Print and shaded views of the part. All mm, measured from the part's lowest x, y and z. A direction names the side the tool comes from. Coordinates: 2 decimals unless noted, no trailing zeros. Order: outer loops, then holes, each group sorted by start corner. A loop starts at its lowest first (then second) coordinate and runs counter-clockwise, first axis right, second up.
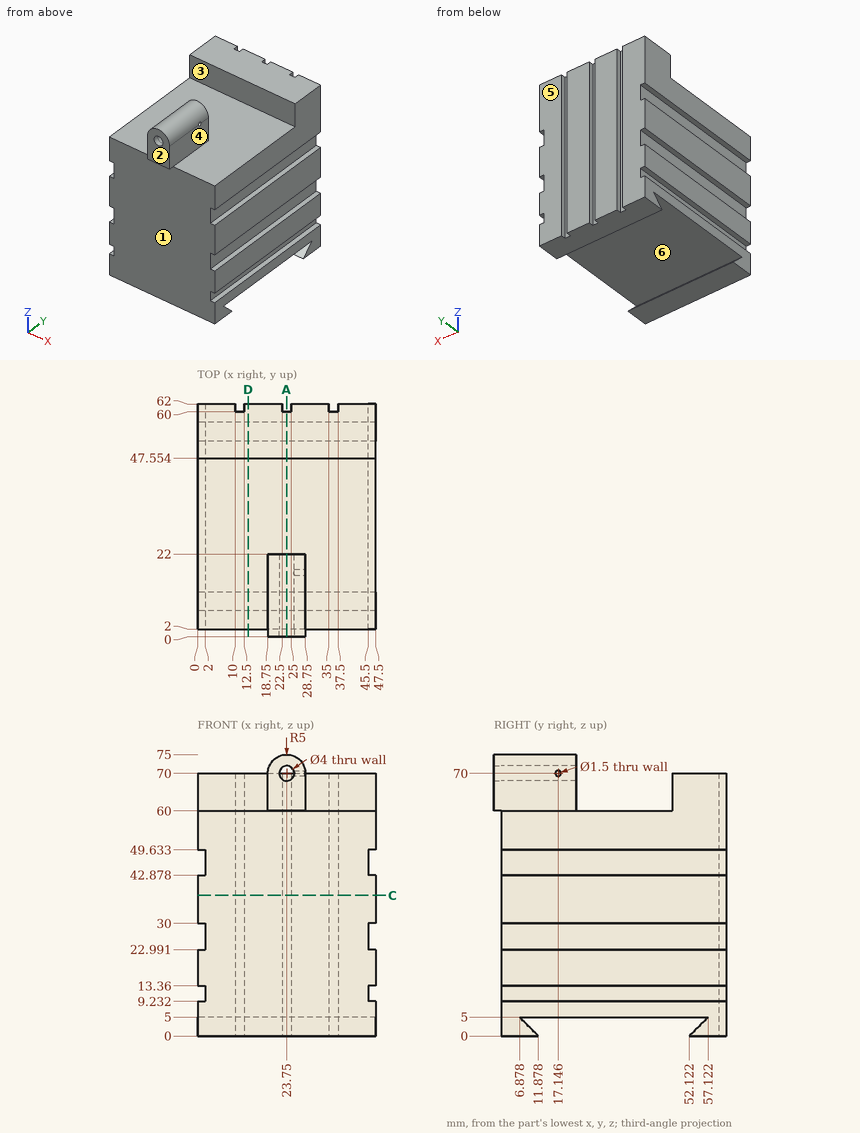
Q1. Cut at D-D, the plane x = 13.5. List the corners of the cut face in (y, z), plus the area to 3 significant figures.
Established:
outline: (2, 0) - (11.88, 0) - (6.88, 5) - (57.12, 5) - (52.12, 0) - (62, 0) - (62, 70) - (47.55, 70) - (47.55, 60) - (2, 60) - close
area: 3,520 mm2
Q2. Probe line 1 (Z direction, x = 23.75, y = 14.75); line 2 (Z direction, x = 23.75, y = 10.25); line 3 (Z direction, x = 23.75, y = 1.65). List the from-to ranges inside material, lowest first.
Established:
line 1: z = 5 to 68, 72 to 75
line 2: z = 0 to 1.63, 5 to 68, 72 to 75
line 3: z = 60 to 68, 72 to 75
Q3. Cut at C-C, the plane z = 37.5. List the corners of the cut face in (x, y).
Established:
outline: (0, 2) - (47.5, 2) - (47.5, 62) - (37.5, 62) - (37.5, 60) - (35, 60) - (35, 62) - (25, 62) - (25, 60) - (22.5, 60) - (22.5, 62) - (12.5, 62) - (12.5, 60) - (10, 60) - (10, 62) - (0, 62) - close
Q4. Mould opens along Y. For the marked faces 4, 5 and 6 say: pulls with the +Y half, pulls with the -Y half, needs draft (parallel to the pull), parting line crosses it, or undercut.
Established:
face 4: needs draft
face 5: pulls with the +Y half
face 6: undercut
Q5. Drop flat-ended pins along their axis: P1, Ø2, axis at y = 17.15, z = 70, coming from the +X side; P2, Ø2, axis at y = 42, z = 29.5, coming from the -X side; P3, Ø0.8, axis at x = 23.5, z = 29.5, coming from the +Y side; P4, Ø2, axis at x = 19, y = 14.5, coming from the +Z side. Give the stop position or say it passes through.
Established:
P1: stops at x = 28.75
P2: stops at x = 0
P3: stops at y = 60
P4: stops at z = 73.31
Q6. Which spindle directions (+Z, -Z, +X, -X, +Y, -Y) get a long thin tool onto all of the face, cutting with end or side? Do the marked faces 1, 2 and 3. Say none if no direction does.
Established:
face 1: -Z, +X, -X, -Y
face 2: +Z, -Z, +X, -X, -Y
face 3: +Z, +X, -X
Q7. Cut at A-A, the plane x = 23.75. List the corners of the cut face in (y, z).
Established:
outline: (0, 60) - (2, 60) - (2, 0) - (11.88, 0) - (6.88, 5) - (57.12, 5) - (52.12, 0) - (60, 0) - (60, 70) - (47.55, 70) - (47.55, 60) - (22, 60) - (22, 68) - (0, 68) - close; (0, 72) - (22, 72) - (22, 75) - (0, 75) - close
